Autodesk Inventor part; units mm, degrees
ref_plane "YZ Plane" through (0, 0, 0) normal (1, 0, 0) x (0, 1, 0)
ref_plane "XZ Plane" through (0, 0, 0) normal (0, 1, 0) x (-1, 0, 0)
ref_plane "XY Plane" through (0, 0, 0) normal (0, 0, 1) x (1, 0, 0)
sketch "Sketch1" plane through (0, 0, 0) normal (0, 1, 0) x (-1, 0, 0)
  line L0 (0, 0) -> (25.4, 0)
  line L1 (25.4, 0) -> (25.4, 50.8)
  line L2 (25.4, 50.8) -> (0, 50.8)
  line L3 (0, 50.8) -> (0, 0)
  line L4 (3.175, 3.175) -> (22.225, 3.175)
  line L5 (22.225, 3.175) -> (22.225, 47.625)
  line L6 (22.225, 47.625) -> (3.175, 47.625)
  line L7 (3.175, 47.625) -> (3.175, 3.175)
  dimension "d0" = 25.4
  dimension "d1" = 50.8
  dimension "d2" = 19.05
  dimension "d3" = 44.45
  dimension "d4" = 3.175
  dimension "d5" = 3.175
extrude "Extrusion1" add sketch "Sketch1" along normal blind 139.7
sketch "Sketch2" plane through (-25.4, 0, 50.8) normal (0, 0, 1) x (1, 0, 0)
  line L0 (0, 0) -> (25.4, 0)
  line L1 (25.4, 0) -> (25.4, 139.7)
  line L2 (0, 139.7) -> (25.4, 139.7)
  line L3 (0, 0) -> (0, 139.7)
  point P0 (12.7, 127)
  point P1 (12.7, 12.7)
  dimension "d8" = 12.7
  dimension "d9" = 12.7
  dimension "d10" = 12.7
  dimension "d11" = 12.7
hole "Hole1" at (-12.7, 127, 50.8) at (-12.7, 12.7, 50.8) direction (0, 0, -1) diameter 6.35 end through all
sketch "Sketch3" plane through (-25.4, 0, 0) normal (-1, 0, 0) x (0, 0, 1)
  line L0 (0, 0) -> (50.8, 0)
  line L1 (50.8, 0) -> (50.8, 139.7)
  line L2 (0, 139.7) -> (50.8, 139.7)
  line L3 (0, 0) -> (0, 139.7)
  circle A0 centre (41.275, 69.85) radius 4.7625 construction
  line L4 (41.275, 69.85) -> (41.275, 65.0875) construction
  line L5 (41.275, 69.85) -> (41.275, 74.6125) construction
  line L6 (50.8, 74.6125) -> (41.275, 74.6125)
  line L7 (50.8, 0) -> (50.8, 139.7)
  line L8 (50.8, 65.0875) -> (41.275, 65.0875)
  line L9 (50.8, 74.6125) -> (50.8, 65.0875)
  arc A1 (41.275, 74.6125) -> (41.275, 65.0875) centre (41.275, 69.85) ccw
  dimension "d19" = 69.85
  dimension "d20" = 9.525
  dimension "d21" = 9.525
extrude "Extrusion2" cut sketch "Sketch3" against normal blind 155.575 contours L8 A1 L6 L1
sketch "Sketch4" plane through (-25.4, 0, 0) normal (-1, 0, 0) x (0, 0, 1)
  line L0 (0, 0) -> (50.8, 0)
  line L1 (0, 0) -> (0, 139.7)
  point P0 (12.7, 63.5)
  point P1 (25.4, 76.2)
  dimension "d24" = 12.7
  dimension "d25" = 12.7
  dimension "d26" = 63.5
  dimension "d27" = 12.7
hole "Hole2" at (-25.4, 63.5, 12.7) at (-25.4, 76.2, 25.4) direction (1, 0, 0) diameter 6.35 end through all
properties part number "2x1 axle support"
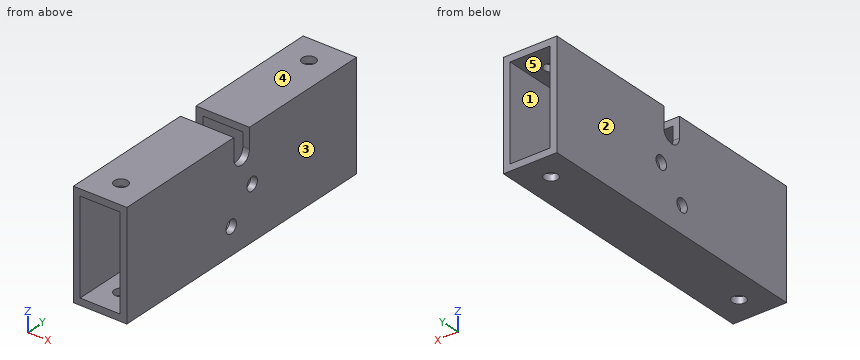
Input: part model. Units: mm. Frame: model coordinates. Face numbers are marked on the shaded views. A direction names the side the tool comes from. Give positions to 0.01 mm unless a question says otherwise; leave off trailing zeros. Order: outer loops, then holes, each group sorted by start corner. A loop starts at its lowest first (then second) coordinate and runs counter-clockwise, first axis right, second up.
1. Set-up query: the marked faces 1 and 2. Return all of +Z, -Z, +X, -X, +Y, -Y with unobstructed straight access to the full face (end or side cutting, diameter ignored); none if empty.
Computed:
face 1: +Y, -Y
face 2: +Z, -Z, -X, +Y, -Y
2. Cut plane C-C (y = 76.2). Return loops of the section in (x, z) (3 decimals).
Computed:
outline: (-25.4, 0) - (0, 0) - (0, 22.225) - (-3.175, 22.225) - (-3.175, 3.175) - (-22.225, 3.175) - (-22.225, 22.225) - (-25.4, 22.225) - close; (-25.4, 28.575) - (-22.225, 28.575) - (-22.225, 47.625) - (-3.175, 47.625) - (-3.175, 28.575) - (0, 28.575) - (0, 50.8) - (-25.4, 50.8) - close
3. Cut plane B-B (x = -12.7). Return loops of the section in (y, z) (1 decimal).
Computed:
outline: (0, 0) - (9.5, 0) - (9.5, 3.2) - (0, 3.2) - close; (0, 47.6) - (9.5, 47.6) - (9.5, 50.8) - (0, 50.8) - close; (15.9, 0) - (123.8, 0) - (123.8, 3.2) - (15.9, 3.2) - close; (15.9, 47.6) - (65.1, 47.6) - (65.1, 50.8) - (15.9, 50.8) - close; (74.6, 47.6) - (123.8, 47.6) - (123.8, 50.8) - (74.6, 50.8) - close; (130.2, 0) - (139.7, 0) - (139.7, 3.2) - (130.2, 3.2) - close; (130.2, 47.6) - (139.7, 47.6) - (139.7, 50.8) - (130.2, 50.8) - close
4. Draft query along Z for the marked faces 3, 4 and 5. Return one class per face: released by +Z, released by -Z, zero draft, split by the parting line, or undercut.
Computed:
face 3: zero draft
face 4: released by +Z
face 5: undercut
5. Cut plane D-D (z = 12.7). Return loops of the section in (x, y) (3 decimals).
Computed:
outline: (-25.4, 0) - (-22.225, 0) - (-22.225, 60.325) - (-25.4, 60.325) - close; (-25.4, 66.675) - (-22.225, 66.675) - (-22.225, 139.7) - (-25.4, 139.7) - close; (-3.175, 0) - (0, 0) - (0, 60.325) - (-3.175, 60.325) - close; (-3.175, 66.675) - (0, 66.675) - (0, 139.7) - (-3.175, 139.7) - close
6. Line query: probe 1 along Y at (x, z) = (-12.7, 2.2) (3 decimals); probe 2 along X at (y, z) = (127, 25.5) (3 decimals); probe 3 along Z at (x, y) = (-6, 91) (3 decimals). Output: solid intervals per line, ascending.
Computed:
probe 1: y = 0 to 9.525, 15.875 to 123.825, 130.175 to 139.7
probe 2: x = -25.4 to -22.225, -3.175 to 0
probe 3: z = 0 to 3.175, 47.625 to 50.8
7. Pin query (flat end, axial travel): pin 1 Ø5.5 at (y, z) = (63.5, 12.7) entering from -X. Return the tip coordinate at first contact, or that it passes through.
Computed:
pin 1: passes through
8. Cut plane A-A (z = 33.5). Return loops of the section in (x, y) (3 decimals), and give its area (3 significant figures).
Computed:
outline: (-25.4, 0) - (-22.225, 0) - (-22.225, 139.7) - (-25.4, 139.7) - close; (-3.175, 0) - (0, 0) - (0, 139.7) - (-3.175, 139.7) - close
area: 887 mm2
